Design review of the part built by this model. Coordinates are the model's own, in mm. A direction names the side the tool comes from. Give positions to 0.01 mm unless a question says otherwise; leave off trailing zeros. Write each loop counter-clockwise with the first axis right and the second up, starting at its lowest first coordinate (ties: lowest second). Pieces come first, ordered by that corner, then holes. Notation, with made-up numbers: (7.5, 82) -> (43.5, 82) arc R25 cw to (43.5, 108) -> close; hole circle Ø3 at (76.5, 55.25). An arc over 180 degrees is marked (long way). Use CSV: the item, a comma, the result in double quotes.
```python
from build123d import *

# Parameters (mm, degrees)
BOX020_W          = 14
BOX020_H          = 6
BOX020_DEPTH      = 20
BOX020_ROLL_ANGLE = 90
BOX021_W          = 14
BOX021_H          = 6
BOX021_DEPTH      = 20
BOX021_ROLL_ANGLE = 90
BOX019_W          = 14
BOX019_H          = 6
BOX019_DEPTH      = 20
BOX019_ROLL_ANGLE = 90
BOX018_W          = 20
BOX018_H          = 30
BOX018_DEPTH      = 25
BOX018_ROLL_ANGLE = 90


with BuildPart() as usb_plug002:
    # Box020 → Box020 (new body)
    with BuildSketch(Plane.XY):
        with Locations((7, 3)):
            Rectangle(BOX020_W, BOX020_H)
    extrude(amount=BOX020_DEPTH)


with BuildPart() as usb_plug002_1:
    # Box020 roll: moved
    add(usb_plug002.part.rotate(Axis((0, 0, 0), (1, 0, 0)), BOX020_ROLL_ANGLE))


with BuildPart() as usb_plug002_2:
    # Box020 placement: moved
    add(usb_plug002_1.part.moved(Location((243, 13, 112))))


with BuildPart() as usb_plug003:
    # Box021 → Box021 (new body)
    with BuildSketch(Plane.XY):
        with Locations((7, 3)):
            Rectangle(BOX021_W, BOX021_H)
    extrude(amount=BOX021_DEPTH)


with BuildPart() as usb_plug003_1:
    # Box021 roll: moved
    add(usb_plug003.part.rotate(Axis((0, 0, 0), (1, 0, 0)), BOX021_ROLL_ANGLE))


with BuildPart() as usb_plug003_2:
    # Box021 placement: moved
    add(usb_plug003_1.part.moved(Location((243, 13, 121))))


with BuildPart() as usb_plug001:
    # Box019 → Box019 (new body)
    with BuildSketch(Plane.XY):
        with Locations((7, 3)):
            Rectangle(BOX019_W, BOX019_H)
    extrude(amount=BOX019_DEPTH)


with BuildPart() as usb_plug001_1:
    # Box019 roll: moved
    add(usb_plug001.part.rotate(Axis((0, 0, 0), (1, 0, 0)), BOX019_ROLL_ANGLE))


with BuildPart() as usb_plug001_2:
    # Box019 placement: moved
    add(usb_plug001_1.part.moved(Location((243, 13, 103))))


with BuildPart() as usb_plug:
    # Box018 → Box018 (new body)
    with BuildSketch(Plane.XY):
        with Locations((10, 15)):
            Rectangle(BOX018_W, BOX018_H)
    extrude(amount=BOX018_DEPTH)


with BuildPart() as usb_plug_1:
    # Box018 roll: moved
    add(usb_plug.part.rotate(Axis((0, 0, 0), (1, 0, 0)), BOX018_ROLL_ANGLE))


with BuildPart() as usb_plug_2:
    # Box018 placement: moved
    add(usb_plug_1.part.moved(Location((240, 20, 100))))

    # Cut012: cut USB Plug001
    add(usb_plug001_2.part, mode=Mode.SUBTRACT)

    # Cut013: cut USB Plug003
    add(usb_plug003_2.part, mode=Mode.SUBTRACT)

    # Cut014: cut USB Plug002
    add(usb_plug002_2.part, mode=Mode.SUBTRACT)


with BuildPart() as usb_plug_3:
    # Cut014 placement: moved
    add(usb_plug_2.part.moved(Location((0, 0, -40))))


solid = usb_plug_3.part
```
(1) Tool access review of faces 5 (the face through (250, 4, 87)), 6 (the face through (240, 8, 75)): name each direction out of +Z, -Z, +X, -X, +Y, -Y from which nothing blocks a thin tool from reaching the whole face with its end or side.
Established:
face 5,"-Y"
face 6,"+Z, -Z, -X, +Y, -Y"
(2) Take a section at B-B (x = 243.5). Write out the cut boundary in (y, z), then the cut area to 3 significant figures.
Established:
outline,"(-5, 60) -> (20, 60) -> (20, 90) -> (-5, 90) -> (-5, 87) -> (13, 87) -> (13, 81) -> (-5, 81) -> (-5, 78) -> (13, 78) -> (13, 72) -> (-5, 72) -> (-5, 69) -> (13, 69) -> (13, 63) -> (-5, 63) -> close"
area,"426 mm2"
(3) For line 1 along Z through (x, y) = (247.25, 9.5); line 2 along X through (y, z) = (2, 85.5); line 3 along Y through (x, z) = (246, 81.75), list the stretches that pass through material, from the lowest coordinate up. Write a range as [from, to].
Established:
line 1,"z = [60, 63], [69, 72], [78, 81], [87, 90]"
line 2,"x = [240, 243], [257, 260]"
line 3,"y = [13, 20]"
(4) Take a section at C-C (z = 82.25). Write out the cut boundary in (x, y).
Established:
outline,"(240, -5) -> (243, -5) -> (243, 13) -> (257, 13) -> (257, -5) -> (260, -5) -> (260, 20) -> (240, 20) -> close"
(5) Take a section at A-A (y = 1.5). Write out the cut boundary in (x, z).
Established:
outline,"(240, 60) -> (260, 60) -> (260, 90) -> (240, 90) -> close; hole (243, 63) -> (257, 63) -> (257, 69) -> (243, 69) -> close; hole (243, 72) -> (257, 72) -> (257, 78) -> (243, 78) -> close; hole (243, 81) -> (257, 81) -> (257, 87) -> (243, 87) -> close"
(6) Mouldability with a two-part tool opening along X and no side actions: class faces 1 (the face through (243, 4, 66)), 2 (the face through (260, 8, 75)), 3 (the face through (257, 4, 84)), 4 (the face through (250, -5, 79)) as +X half, -X half, draft (parallel to the pull), parting line (faces both ways), or undercut.
Established:
face 1,"undercut"
face 2,"+X half"
face 3,"undercut"
face 4,"draft"
(7) Clearance check with a flat-ended pin moving along its axis: pin 1 (1.5 mm diameter, centred on x = 253.5, z = 77, fed in from -Y). State where the tip first meets the part, or that it passes through.
Established:
pin 1,"stops at y = 13"
